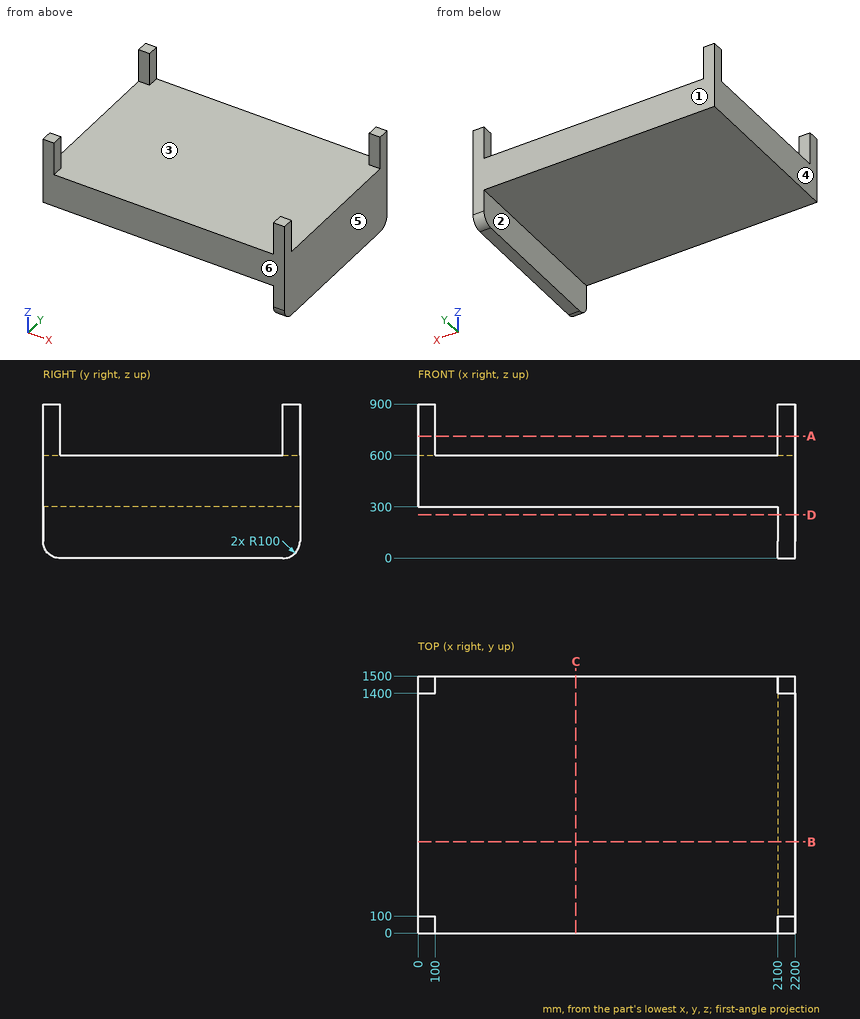
Verification items for this drawing (mm, ordinates from the low corner). A direction names the side the tool comes from. Give positions to 0.01 mm unless a question says otherwise; leave off trailing zeros. Write each loop counter-clockwise with the first axis right and the second up, starting at its lowest first coordinate (ties: lowest second). Pieces come first, ordered by that corner, then holes.
1) Go/stop test with a flat-tipped pin: pin 1 Ø8 at (x, y) = (1500.5, 1242) entering from +Z. Record where the tip stops, or that it passes through.
Values follow:
pin 1: stops at z = 600
2) Thickness scan on line 1 (X direction, y = 366, z = 38); line 2 (X direction, y = 1417, z = 685); line 3 (Z direction, x = 486, y = 733). Record the ranges inside material, lowest first.
Values follow:
line 1: x = 2100 to 2200
line 2: x = 0 to 100, 2100 to 2200
line 3: z = 300 to 600
3) Cross-section at A-A (z = 713). Record the boundary of the cut face in (x, y), plus the area to 3 significant figures.
Values follow:
outline: (0, 0) - (100, 0) - (100, 100) - (0, 100) - close; (0, 1400) - (100, 1400) - (100, 1500) - (0, 1500) - close; (2100, 0) - (2200, 0) - (2200, 100) - (2100, 100) - close; (2100, 1400) - (2200, 1400) - (2200, 1500) - (2100, 1500) - close
area: 40,000 mm2
4) Cross-section at C-C (x = 921). Record the boundary of the cut face in (y, z), plus the area to 3 significant figures.
Values follow:
outline: (0, 300) - (1500, 300) - (1500, 600) - (0, 600) - close
area: 450,000 mm2
5) Cross-section at D-D (z = 253.5). Record the boundary of the cut face in (x, y).
Values follow:
outline: (2100, 0) - (2200, 0) - (2200, 1500) - (2100, 1500) - close
6) Cross-section at B-B (y = 533). Record the boundary of the cut face in (x, z), plus the area to 3 significant figures.
Values follow:
outline: (0, 300) - (2100, 300) - (2100, 0) - (2200, 0) - (2200, 600) - (0, 600) - close
area: 690,000 mm2
7) Set-up check for the marked faces 1 and 2: record each of +Z, -Z, +X, -X, +Y, -Y from which the full face is reachable in a straight line by a thin tool's end or side.
Values follow:
face 1: +Z, -Z, +X, -X, +Y
face 2: -Z, -X, +Y, -Y
8) Release check for a two-part mould opening along X. For the marked faces 3, 4, 5 and 6 record: released by +X, released by -X, zero draft, split by the parting line, or undercut.
Values follow:
face 3: undercut
face 4: released by -X
face 5: released by +X
face 6: zero draft
